from build123d import *

# Parameters (mm, degrees)
SKETCH_1_W           = 58
SKETCH_1_H           = 10
EXTRUDE_1_DEPTH      = 1
HOLE_WIZARD_M3_1_D   = 3.2
HOLE_WIZARD_M3_1_2_D = 3


with BuildPart() as part:
    # 草图1 → 凸台-拉伸1 (new body)
    with BuildSketch(Plane(origin=(0, 0, 0), x_dir=(0, 0, -1), z_dir=(1, 0, 0))):
        Rectangle(SKETCH_1_W, SKETCH_1_H)
    extrude(amount=EXTRUDE_1_DEPTH)

    # Hole Wizard M3 _1 (through all)
    with Locations(Plane(origin=(1, 0, 0), x_dir=(0, 0, -1), z_dir=(1, 0, 0))):
        with Locations((16, 0), (0, 0)):
            Hole(HOLE_WIZARD_M3_1_D / 2)

    # Hole Wizard M3 _1 2 (through all)
    with Locations(Plane(origin=(1, 0, 0), x_dir=(0, 0, -1), z_dir=(1, 0, 0))):
        with Locations((25, 0)):
            Hole(HOLE_WIZARD_M3_1_2_D / 2)


solid = part.part
Verification items for the finished model (mm, model axes). Give positions to 0.01 mm unless a question says otherwise; leave off trailing zeros. Write each loop counter-clockwise with the first axis right and the second up, starting at its lowest first coordinate (ties: lowest second). Pieces come first, ordered by that corner, then holes. Notation, with made-up numbers: M 15.5,9.5 L 57.5,9.5 A13 ccw 57.5,17.5 Z; hole C -23,37 d2. An arc over 180 degrees is marked long. Use CSV: the item, a comma, the result in double quotes.
1) Cross-section at C-C (x = 0.85). Enter the section's corners in (y, z).
Final values:
outline,"M -5,-29 L 5,-29 L 5,29 L -5,29 Z; hole C 0,-16 d3.2; hole C 0,0 d3.2; hole C 0,-25 d3"
2) Cross-section at D-D (z = 0). Enter the section's corners in (x, y), plus the area to 3 significant figures.
Final values:
outline,"M 0,-5 L 1,-5 L 1,-1.6 L 0,-1.6 Z; M 0,1.6 L 1,1.6 L 1,5 L 0,5 Z"
area,"6.80 mm²"
3) Go/stop test with a flat-tipped pin: pin 1 Ø2.5 at (y, z) = (0, -16) entering from -X. Record where the tip stops, or that it passes through.
Final values:
pin 1,"through"
4) Release check for a two-part mould opening along Y. For faces 1 (the face through (0.49, -0.97, -1.27)), 2 (the face through (0, 2, 0)), 3 (the face through (0.5, 5, 0.4)) record: released by +Y, released by -Y, zero draft, split by the parting line, or undercut.
Final values:
face 1,"undercut"
face 2,"zero draft"
face 3,"released by +Y"
5) Cross-section at A-A (y = 0). Enter the section's corners in (x, z).
Final values:
outline,"M 0,-29 L 1,-29 L 1,-26.5 L 0,-26.5 Z; M 0,-23.5 L 1,-23.5 L 1,-17.6 L 0,-17.6 Z; M 0,-14.4 L 1,-14.4 L 1,-1.6 L 0,-1.6 Z; M 0,1.6 L 1,1.6 L 1,29 L 0,29 Z"
6) Cross-section at B-B (z = -25). Enter the section's corners in (x, y), plus the area to 3 significant figures.
Final values:
outline,"M 0,-5 L 1,-5 L 1,-1.5 L 0,-1.5 Z; M 0,1.5 L 1,1.5 L 1,5 L 0,5 Z"
area,"7.00 mm²"
7) Material ranges on line 1 along Y through (x, z) = (0.5, -25); line 2 along Y through (x, z) = (0.6, -16), recorded low to high.
Final values:
line 1,"-5 to -1.5, 1.5 to 5"
line 2,"-5 to -1.6, 1.6 to 5"
